Could you check a few things on this drawing? It's one solid part, dimensions in mm from its lowest x, y, z. A direction names the side the tool comes from. Round coordinates to 2 decimals unless told otherwise and drop trailing zeros. Loops run counter-clockwise (first coordinate to the right, second up) from the corner with the lowest first, then second, coordinate; pieces in that order, holes last. Notation, with made-up numbers: M 40,-15.75 L 69,-15.75 A22 cw 69,4.25 Z; hole C 78.5,4.5 d10. An arc over 180 degrees is marked long. Answer as CSV lines item,"result".
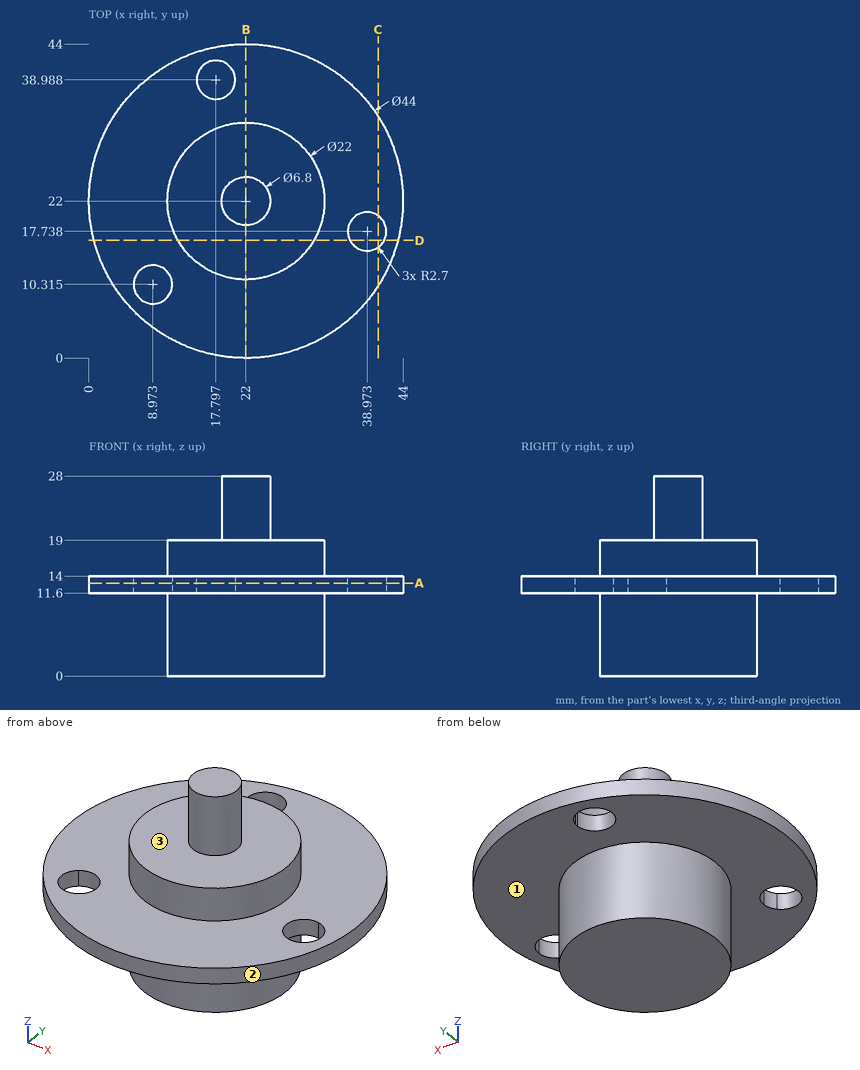
Item 1: If we section it at B-B on x = 22: Write out the boundary of the cut face in (y, z).
Output:
outline,"M 0,11.6 L 11,11.6 L 11,0 L 33,0 L 33,11.6 L 44,11.6 L 44,14 L 33,14 L 33,19 L 25.4,19 L 25.4,28 L 18.6,28 L 18.6,19 L 11,19 L 11,14 L 0,14 Z"
Item 2: Will these pins go through, and if not, where does the flat tip stop? pin 1 (1.5 mm diameter, centred on x = 5, z = 11.5, fed in from -Y); pin 2 (10 mm diameter, centred on x = 16.5, y = 5, fed in from -Z); pin 3 (3 mm diameter, centred on x = 29, z = 19, fed in from +Y).
Output:
pin 1,"stops at y = 7.18"
pin 2,"stops at z = 11.6"
pin 3,"stops at y = 31.53"
Item 3: If we section it at C-C on x = 40.5: Write out the boundary of the cut face in (y, z) (1 decimal).
Output:
outline,"M 10.1,11.6 L 15.5,11.6 L 15.5,14 L 10.1,14 Z; M 20,11.6 L 33.9,11.6 L 33.9,14 L 20,14 Z"
Item 4: If we section it at D-D on y = 16.5: Write out the boundary of the cut face in (x, z), then the cut area to 3 significant figures.
Output:
outline,"M 0.7,11.6 L 12.47,11.6 L 12.47,0 L 31.53,0 L 31.53,11.6 L 36.57,11.6 L 36.57,14 L 31.53,14 L 31.53,19 L 12.47,19 L 12.47,14 L 0.7,14 Z; M 41.37,11.6 L 43.3,11.6 L 43.3,14 L 41.37,14 Z"
area,"407 mm2"
Item 5: If we section it at A-A on z = 13: State how many separate pieces and enclosed holes the cut face has, then the cut area to 3 significant figures.
Output:
separate pieces,"1"
enclosed holes,"3"
area,"1,450 mm2"
Item 6: On a 3-axis mill with a long thin cutter (end or side, diameter ignored), from which of +Z, -Z, +X, -X, +Y, -Y can I reach the whole of each face in a straight line? I mean the marked faces 1, 2 and 3. Say none if no direction works.
Output:
face 1,"-Z"
face 2,"+Z, -Z"
face 3,"+Z"
Item 7: If I drill on line 1 along Z through (x, y) = (10, 21); line 2 along Z through (x, y) = (31.5, 20); line 3 along Y through (x, z) = (25.5, 2.5), over which ranges is the centre line in solid material (lowest first)? Write a range as from..to.
Output:
line 1,"z = 11.6..14"
line 2,"z = 0..19"
line 3,"y = 11.57..32.43"
